Check sheet for the modelled part. Datum: model origin and axes. Units: mm. A direction names the side the tool comes from. Round coordinates to 2 decimals unless told otherwise and drop trailing zeros. Loops run counter-clockwise (first coordinate to the right, second up) from the corner with the lowest first, then second, coordinate; pieces in that order, holes last. Notation, with made-up numbers: (87, 24) - (113, 24) arc R36 ccw to (113, 58) - close; hole circle Ø4 at (-25, 19.25). An arc over 180 degrees is marked (long way). Return JSON: item names as keys, results as strings.
from build123d import *

# Parameters (mm, degrees)
BOSS_EXTRUDE1_DEPTH     = 31
SKETCH5_W               = 21
SKETCH5_H               = 70
CUT_EXTRUDE3_DEPTH      = 110
SKETCH6_R               = 6
CUT_EXTRUDE4_DEPTH      = 110
SKETCH7_W               = 82.876057885
SKETCH7_H               = 21.558852062
CUT_EXTRUDE5_DEPTH      = 110
CUT_EXTRUDE6_DEPTH      = 116.208083877
CUT_EXTRUDE6_DEPTH_BACK = 116.208083877
SKETCH8_R               = 13.04144487


with BuildPart() as part:
    # Sketch1 → Boss-Extrude1 (new body)
    with BuildSketch(Plane.XY):
        Polygon((-75.552372261, 34.084409915), (-75.552372261, -65.915590085), (-5.552372261, -65.915590085), (-33.28739918, 34.084409915), align=None)
    extrude(amount=BOSS_EXTRUDE1_DEPTH)

    # Sketch5 → Cut-Extrude3 (cut)
    with BuildSketch(Plane.ZY.offset(75.552372261)):
        with Locations((15.5, -25.915590085)):
            Rectangle(SKETCH5_W, SKETCH5_H)
    extrude(amount=-CUT_EXTRUDE3_DEPTH, mode=Mode.SUBTRACT)

    # Sketch6 → Cut-Extrude4 (cut)
    with BuildSketch(Plane(origin=(0, -60.915590085, 0), x_dir=(1, 0, 0), z_dir=(0, 1, 0))):
        with Locations(Location((-60.552372261, -14.649638942, 0), (0, 0, 270))):
            Circle(SKETCH6_R)
    extrude(amount=-CUT_EXTRUDE4_DEPTH, mode=Mode.SUBTRACT)

    # Sketch7 → Cut-Extrude5 (cut)
    with BuildSketch(Plane.ZY.offset(75.552372261)):
        with Locations((20.394948081, 24.863835946)):
            Rectangle(SKETCH7_W, SKETCH7_H)
    extrude(amount=-CUT_EXTRUDE5_DEPTH, mode=Mode.SUBTRACT)

    # Sketch8 → Cut-Extrude6 (cut, two sides: drawn at the far end of the back side and taken through both)
    with BuildSketch(Plane(origin=(-5.60875104, 20.222626991, 0), x_dir=(0.9636240692030443, 0.2672613949910582, 0), z_dir=(-0.2672613949910583, 0.9636240692030444, 0)).offset(-CUT_EXTRUDE6_DEPTH_BACK)):
        with Locations((-22.96709211, -15.5)):
            Circle(SKETCH8_R)
    extrude(amount=CUT_EXTRUDE6_DEPTH + CUT_EXTRUDE6_DEPTH_BACK, mode=Mode.SUBTRACT)


solid = part.part
Q1. Sectioned sample at A-A (x = -43). Enter the section's corners in (y, z).
Answer key:
{"outline": "(-65.92, 0) - (14.08, 0) - (14.08, 31) - (-65.92, 31) - close; hole (-60.92, 5) - (9.08, 5) - (9.08, 26) - (-60.92, 26) - close"}
Q2. Sectioned sample at C-C (z = 14.5). Enter the section's corners in (x, y).
Answer key:
{"outline": "(-75.55, -65.92) - (-66.55, -65.92) - (-66.55, -60.92) - (-75.55, -60.92) - close; (-75.55, 9.08) - (-39.85, 9.08) - (-41.23, 14.08) - (-75.55, 14.08) - close; (-54.55, -65.92) - (-19.05, -65.92) - (-20.43, -60.92) - (-54.55, -60.92) - close"}
Q3. Depth check by flat-ended pin: P1, Ø10.5, axis at x = -59, z = 11.5, coming from the -Y side. Enter the tip coordinate at first touch or a pass-through.
Answer key:
{"P1": "stops at y = -65.92"}
Q4. Sectioned sample at B-B (z = 19). Enter the section's corners in (x, y).
Answer key:
{"outline": "(-75.55, -65.92) - (-64.68, -65.92) - (-64.68, -60.92) - (-75.55, -60.92) - close; (-75.55, 9.08) - (-39.39, 9.08) - (-40.78, 14.08) - (-75.55, 14.08) - close; (-56.42, -65.92) - (-18.59, -65.92) - (-19.98, -60.92) - (-56.42, -60.92) - close"}
Q5. Draft check along Z on faces 4 (the face through (-49, -25, 0)), 5 (the face through (-23.01, -26.433, 4.065)), 6 (the face through (-57, 14.084, 15)). Enter one of: released by +Z, released by -Z, zero draft, split by the parting line, or undercut.
Answer key:
{"face 4": "released by -Z", "face 5": "undercut", "face 6": "zero draft"}
Q6. Scan lines: probe 1 along Z at (x, y) = (-55.5, -49.5); probe 2 along Y at (x, z) = (-41.5, 18); probe 3 along Y at (x, z) = (-33, 19). Record each from-to range of solid material in increasing order. Write a range as [from, to].
Answer key:
{"probe 1": "z = [0, 5], [26, 31]", "probe 2": "y = [-65.92, -60.92], [9.08, 14.08]", "probe 3": "y = [-65.92, -60.92]"}
Q7. Tool access check on faces 1 (the face through (-41, -65.916, 15)), 2 (the face through (-56.497, -63.381, 10.227)), 3 (the face through (-55, 9.084, 15)). Record the directions out of +Z, -Z, +X, -X, +Y, -Y that give a thin tool (end or side, any length) a straight path to the whole face; none if there is none.
Answer key:
{"face 1": "+Z, -Z, +X, -X, -Y", "face 2": "-Y", "face 3": "+X, -X"}
